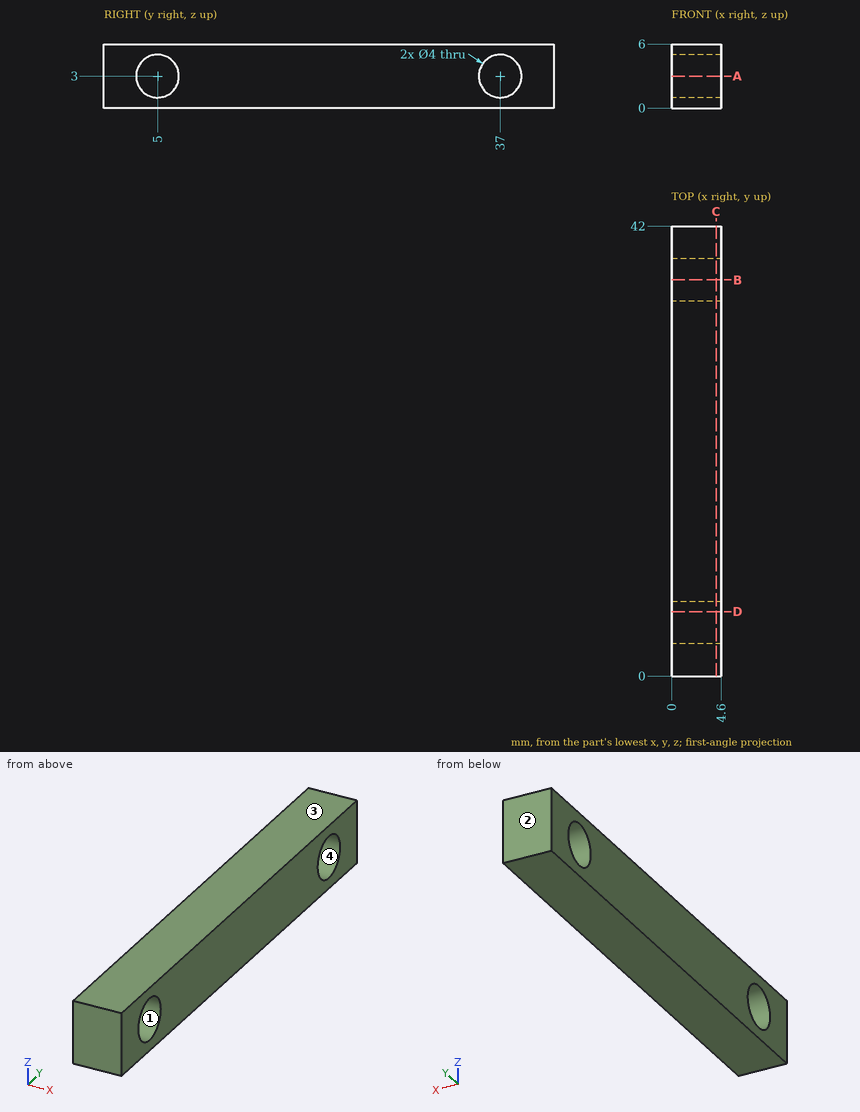
Input: dimensioned drawing with shaded views. Units: mm. Origin: part minimum x, y, z. Give positions to 0.01 mm unless a question says otherwise; leave off trailing zeros. Write each loop counter-clockwise with the first axis right and the second up, starting at its lowest first coordinate (ties: lowest second). Pieces come first, ordered by that corner, then holes.
1. Section query B-B, the plane y = 37. Return loops of the section in (x, z).
2. Section query C-C, the plane x = 4.15. Return loops of the section in (y, z).
3. Draft query along Y for the marked faces 1, 2, 3 and 4. Return one class per face: released by +Y, released by -Y, zero draft, split by the parting line, or undercut.
4. Section query D-D, the plane y = 6. Return loops of the section in (x, z).
5. Pin query (flat end, axial travel): P1, Ø2.5, axis at y = 37, z = 3, coming from the -X side. Return the tip coordinate at first contact, or that it passes through.
6. Section query A-A, the plane z = 3. Return loops of the section in (x, y).
7. Line query: probe 1 along Y at (x, z) = (0.75, 3.1); probe 2 along Y at (x, z) = (2.9, 2.15); probe 3 along Z at (x, y) = (2.1, 5). Output: solid intervals per line, ascending.
Computed:
1. outline: (0, 0) - (4.6, 0) - (4.6, 1) - (0, 1) - close; (0, 5) - (4.6, 5) - (4.6, 6) - (0, 6) - close
2. outline: (0, 0) - (42, 0) - (42, 6) - (0, 6) - close; hole circle Ø4 at (5, 3); hole circle Ø4 at (37, 3)
3. face 1: undercut
3. face 2: released by +Y
3. face 3: zero draft
3. face 4: undercut
4. outline: (0, 0) - (4.6, 0) - (4.6, 1.27) - (0, 1.27) - close; (0, 4.73) - (4.6, 4.73) - (4.6, 6) - (0, 6) - close
5. P1: passes through
6. outline: (0, 0) - (4.6, 0) - (4.6, 3) - (0, 3) - close; (0, 7) - (4.6, 7) - (4.6, 35) - (0, 35) - close; (0, 39) - (4.6, 39) - (4.6, 42) - (0, 42) - close
7. probe 1: y = 0 to 3, 7 to 35, 39 to 42
7. probe 2: y = 0 to 3.19, 6.81 to 35.19, 38.81 to 42
7. probe 3: z = 0 to 1, 5 to 6
